```python
from build123d import *

# Parameters (mm, degrees)
SKETCH1_W          = 80
SKETCH1_H          = 212.4467896
SKETCH1_W_2        = 10
SKETCH1_H_2        = 50
SKETCH1_H_3        = 30
BASE_FLANGE1_DEPTH = 2


# Sheet-metal steps are written as plain solids
with BuildPart() as part:
    # Sketch1 → Base-Flange1 (new body)
    with BuildSketch(Plane(origin=(0, 0, 0), x_dir=(0, 0, -1), z_dir=(1, 0, 0))):
        with Locations((-40, 106.2233948)):
            Rectangle(SKETCH1_W, SKETCH1_H)
        with Locations((-65, 177.4467896)):
            Rectangle(SKETCH1_W_2, SKETCH1_H_2, mode=Mode.SUBTRACT)
        with Locations((-35, 177.4467896)):
            Rectangle(SKETCH1_W_2, SKETCH1_H_2, mode=Mode.SUBTRACT)
        with Locations((-15, 177.4467896)):
            Rectangle(SKETCH1_W_2, SKETCH1_H_2, mode=Mode.SUBTRACT)
        with Locations((-60, 25)):
            Rectangle(SKETCH1_W_2, SKETCH1_H_3, mode=Mode.SUBTRACT)
        with Locations((-40, 25)):
            Rectangle(SKETCH1_W_2, SKETCH1_H_3, mode=Mode.SUBTRACT)
    extrude(amount=-BASE_FLANGE1_DEPTH)


solid = part.part
```
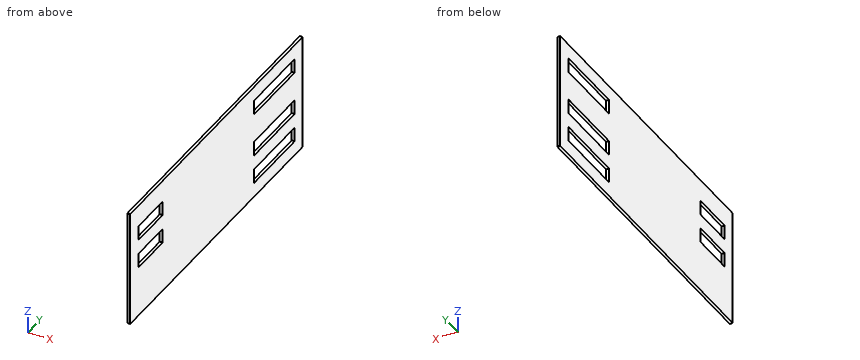
Design review of the part built by this model. Coordinates are the model's own, in mm. Coordinates: 2 decimals unless noted, no trailing zeros. Order: outer loops, then holes, each group sorted by start corner. A loop starts at its lowest first (then second) coordinate and runs counter-clockwise, first axis right, second up. Notation, with made-up numbers: (38.5, 28.5) -> (73.5, 28.5) arc R20 cw to (73.5, 41.5) -> close; hole circle Ø2 at (-23.5, 88). An arc over 180 degrees is marked (long way). One line per item, written item: value. Start each with the question number.
Q1. For probe 1 along Z at (x, y) = (-1.45, 189); probe 2 along Z at (x, y) = (-0.8, 39); probe 3 along Y at (x, z) = (-0.3, 37.5), list the stretches that pass through material, from the lowest coordinate up.
Q2. Take a section at B-B, the plane z = 15.5. State the section outline as (x, y) points, then the cut area to 3 significant figures.
Q3. Take a section at D-D, the plane y = 36. State the section outline as (x, z) points, then the cut area to 3 significant figures.
Q4. Take a section at C-C, the plane x = -1.3. State the section outline as (y, z) points.
Q5. Take a section at A-A, the plane y = 180.5. State the section outline as (x, z) points, then the cut area to 3 significant figures.
Values follow:
1. probe 1: z = 0 to 10, 20 to 30, 40 to 60, 70 to 80
1. probe 2: z = 0 to 35, 45 to 55, 65 to 80
1. probe 3: y = 0 to 10, 40 to 152.45, 202.45 to 212.45
2. outline: (-2, 0) -> (0, 0) -> (0, 152.45) -> (-2, 152.45) -> close; (-2, 202.45) -> (0, 202.45) -> (0, 212.45) -> (-2, 212.45) -> close
2. area: 325 mm2
3. outline: (-2, 0) -> (0, 0) -> (0, 35) -> (-2, 35) -> close; (-2, 45) -> (0, 45) -> (0, 55) -> (-2, 55) -> close; (-2, 65) -> (0, 65) -> (0, 80) -> (-2, 80) -> close
3. area: 120 mm2
4. outline: (0, 0) -> (212.45, 0) -> (212.45, 80) -> (0, 80) -> close; hole (10, 35) -> (40, 35) -> (40, 45) -> (10, 45) -> close; hole (10, 55) -> (40, 55) -> (40, 65) -> (10, 65) -> close; hole (152.45, 10) -> (202.45, 10) -> (202.45, 20) -> (152.45, 20) -> close; hole (152.45, 30) -> (202.45, 30) -> (202.45, 40) -> (152.45, 40) -> close; hole (152.45, 60) -> (202.45, 60) -> (202.45, 70) -> (152.45, 70) -> close
5. outline: (-2, 0) -> (0, 0) -> (0, 10) -> (-2, 10) -> close; (-2, 20) -> (0, 20) -> (0, 30) -> (-2, 30) -> close; (-2, 40) -> (0, 40) -> (0, 60) -> (-2, 60) -> close; (-2, 70) -> (0, 70) -> (0, 80) -> (-2, 80) -> close
5. area: 100 mm2
